```python
from build123d import *

# Parameters (mm, degrees)
ESQUISSE1_W             = 199
ESQUISSE1_H             = 48
BOSS_EXTRU_1_DEPTH      = 6
ESQUISSE2_W             = 20
ESQUISSE2_H             = 6
BOSS_EXTRU_2_DEPTH      = 6
ESQUISSE3_W             = 6
ESQUISSE3_H             = 20
BOSS_EXTRU_3_DEPTH      = 6
ESQUISSE4_W             = 78
ESQUISSE4_H             = 5
ENL_V_MAT_EXTRU_1_DEPTH = 213.077815907
ENL_V_MAT_EXTRU_2_DEPTH = 213.077815907
ESQUISSE6_R             = 1.005
ENL_V_MAT_EXTRU_3_DEPTH = 213.077815907
ESQUISSE7_R             = 2
ENL_V_MAT_EXTRU_4_DEPTH = 3


with BuildPart() as part:
    # Esquisse1 → Boss.-Extru.1 (new body)
    with BuildSketch(Plane.XY):
        with Locations((-99.5, 24)):
            Rectangle(ESQUISSE1_W, ESQUISSE1_H)
    extrude(amount=BOSS_EXTRU_1_DEPTH)

    # Esquisse2 → Boss.-Extru.2 (add)
    with BuildSketch(Plane(origin=(0, 48, 0), x_dir=(1, 0, 0), z_dir=(0, 1, 0))):
        with Locations((-99, -3)):
            Rectangle(ESQUISSE2_W, ESQUISSE2_H)
        with Locations((-159, -3)):
            Rectangle(ESQUISSE2_W, ESQUISSE2_H)
    extrude(amount=BOSS_EXTRU_2_DEPTH)

    # Esquisse3 → Boss.-Extru.3 (add)
    with BuildSketch(Plane.ZY.offset(199)):
        with Locations((3, 24)):
            Rectangle(ESQUISSE3_W, ESQUISSE3_H)
    extrude(amount=BOSS_EXTRU_3_DEPTH)

    # Esquisse4 → Enlèv. mat.-Extru.1 (cut, through all)
    with BuildSketch(Plane.XY.offset(6)):
        with Locations((-39, 2.5)):
            Rectangle(ESQUISSE4_W, ESQUISSE4_H)
    extrude(amount=-ENL_V_MAT_EXTRU_1_DEPTH, mode=Mode.SUBTRACT)

    # Esquisse5 → Enlèv. mat.-Extru.2 (cut, through all)
    with BuildSketch(Plane.XY.offset(6)):
        Polygon((0, 48), (-40, 48), (0, 5), align=None)
    extrude(amount=-ENL_V_MAT_EXTRU_2_DEPTH, mode=Mode.SUBTRACT)

    # Esquisse6 → Enlèv. mat.-Extru.3 (cut, through all)
    with BuildSketch(Plane.XY.offset(6)):
        with Locations((-148.88, 14.5)):
            Circle(ESQUISSE6_R)
        with Locations((-148.88, 30.5)):
            Circle(ESQUISSE6_R)
        with Locations((-132.88, 14.5)):
            Circle(ESQUISSE6_R)
        with Locations((-132.88, 30.5)):
            Circle(ESQUISSE6_R)
        with Locations((-116.88, 14.5)):
            Circle(ESQUISSE6_R)
        with Locations((-116.88, 30.5)):
            Circle(ESQUISSE6_R)
        with Locations((-100.88, 14.5)):
            Circle(ESQUISSE6_R)
        with Locations((-100.88, 30.5)):
            Circle(ESQUISSE6_R)
        with Locations((-84.88, 14.5)):
            Circle(ESQUISSE6_R)
        with Locations((-84.88, 30.5)):
            Circle(ESQUISSE6_R)
        with Locations((-68.88, 14.5)):
            Circle(ESQUISSE6_R)
        with Locations((-68.88, 30.5)):
            Circle(ESQUISSE6_R)
        with Locations((-52.88, 14.5)):
            Circle(ESQUISSE6_R)
        with Locations((-52.88, 30.5)):
            Circle(ESQUISSE6_R)
        with Locations((-164.88, 14.5)):
            Circle(ESQUISSE6_R)
        with Locations((-164.88, 30.5)):
            Circle(ESQUISSE6_R)
        with Locations((-180.88, 14.5)):
            Circle(ESQUISSE6_R)
        with Locations((-180.88, 30.5)):
            Circle(ESQUISSE6_R)
    extrude(amount=-ENL_V_MAT_EXTRU_3_DEPTH, mode=Mode.SUBTRACT)

    # Esquisse7 → Enlèv. mat.-Extru.4 (cut)
    with BuildSketch(Plane(origin=(0, 0, 0), x_dir=(-1, 0, 0), z_dir=(0, 0, -1))):
        with Locations((180.88, 14.5)):
            Circle(ESQUISSE7_R)
        with Locations((180.88, 30.5)):
            Circle(ESQUISSE7_R)
        with Locations((164.88, 14.5)):
            Circle(ESQUISSE7_R)
        with Locations((164.88, 30.5)):
            Circle(ESQUISSE7_R)
        with Locations((148.88, 14.5)):
            Circle(ESQUISSE7_R)
        with Locations((148.88, 30.5)):
            Circle(ESQUISSE7_R)
        with Locations((132.88, 14.5)):
            Circle(ESQUISSE7_R)
        with Locations((132.88, 30.5)):
            Circle(ESQUISSE7_R)
        with Locations((116.88, 14.5)):
            Circle(ESQUISSE7_R)
        with Locations((116.88, 30.5)):
            Circle(ESQUISSE7_R)
        with Locations((100.88, 14.5)):
            Circle(ESQUISSE7_R)
        with Locations((100.88, 30.5)):
            Circle(ESQUISSE7_R)
        with Locations((84.88, 14.5)):
            Circle(ESQUISSE7_R)
        with Locations((84.88, 30.5)):
            Circle(ESQUISSE7_R)
        with Locations((68.88, 14.5)):
            Circle(ESQUISSE7_R)
        with Locations((68.88, 30.5)):
            Circle(ESQUISSE7_R)
        with Locations((52.88, 14.5)):
            Circle(ESQUISSE7_R)
        with Locations((52.88, 30.5)):
            Circle(ESQUISSE7_R)
    extrude(amount=-ENL_V_MAT_EXTRU_4_DEPTH, mode=Mode.SUBTRACT)


solid = part.part
```
CAD build for the part. Positions are in the model's coordinates, mm. A direction names the side the tool comes from. Round coordinates to 2 decimals unless told otherwise and drop trailing zeros. Write each loop counter-clockwise with the first axis right and the second up, starting at its lowest first coordinate (ties: lowest second). Pieces come first, ordered by that corner, then holes. Notation, with made-up numbers: (60, -17) - (71, -17) arc R32 ccw to (71, 16) - close; hole circle Ø1 at (-36.5, 50.5). An arc over 180 degrees is marked (long way). Return JSON: item names as keys, results as strings. Group by question number.
Item 1: Band-saw the part on B-B on x = -123.5. List the corners of the cut face in (y, z).
Item 2: Band-saw the part on A-A on z = 1.3. State how many separate pieces and enclosed holes the cut face has, plus the area to 3 significant figures.
Item 3: 3-axis set-ups, long thin cutter, end or side, ignore diameter. For faces 4 (the face through (-109, 51, 3)), 5 (the face through (-70.727, 29.734, 1.479)), 6 (the face through (-199, 41, 3)), 7 (the face through (-202, 14, 3)): which of +Z, -Z, +X, -X, +Y, -Y reach the whole face in a straight line?
Item 4: Band-saw the part on C-C on y = 38. List the corners of the cut face in (x, z).
Item 5: Flat gauge pins, fed straight in: pin 1 Ø1.2 at (x, y) = (-132.88, 30.5) entering from -Z; pin 2 Ø2.5 at (x, y) = (-52.88, 30.5) entering from -Z; pin 3 Ø3 at (x, y) = (-68.88, 30.5) entering from +Z; pin 4 Ø1.5 at (x, z) = (-42.5, 5.5) entering from +Y. Where does each tip first touch, or does it go through?
Item 6: Mould opens along Y. For faces 1 (the face through (-89, 51, 3)), 2 (the face through (-86.727, 29.734, 1.479)), 3 (the face through (-202, 34, 3)) say: +Y half, -Y half, draft (parallel to the pull), parting line (faces both ways), or undercut.
Item 7: Probe probe 1 along Y at (x, z) = (-116.88, 0.95); probe 2 along Y at (x, z) = (-164.88, 4.4) (3 decimals); probe 3 along X at (y, z) = (48.5, 2.6). List the from-to ranges inside material, lowest first.
Resolved:
{
 "1": {"outline": "(0, 0) - (48, 0) - (48, 6) - (0, 6) - close"},
 "2": {"separate pieces": "1", "enclosed holes": "18", "area": "8,440 mm²"},
 "3": {"face 4": "+Z, -Z, +Y", "face 5": "-Z", "face 6": "+Z, -Z, -X, +Y", "face 7": "+Z, -Z, -X, -Y"},
 "4": {"outline": "(-199, 0) - (-30.7, 0) - (-30.7, 6) - (-199, 6) - close"},
 "5": {"pin 1": "passes through", "pin 2": "stops at z = 3", "pin 3": "stops at z = 6", "pin 4": "stops at y = 48"},
 "6": {"face 1": "draft", "face 2": "undercut", "face 3": "+Y half"},
 "7": {"probe 1": "y = 0 to 12.5, 16.5 to 28.5, 32.5 to 48", "probe 2": "y = 0 to 13.495, 15.505 to 29.495, 31.505 to 54", "probe 3": "x = -169 to -149, -109 to -89"}
}
